from build123d import *

# Parameters (mm, degrees)
BOSS_EXTRUDE1_DEPTH = 3.302


with BuildPart() as part:
    # Sketch2 → Revolve1 (revolve)
    with BuildSketch(Plane(origin=(0, 0, 0), x_dir=(0, 0, -1), z_dir=(1, 0, 0)), mode=Mode.PRIVATE) as revolve1_sk:
        Polygon((0, 3.556), (-4.2672, 3.556), (-4.2672, 5.08), (-7.366, 5.08), (-28.702, 3.8735), (-28.702, 3.556), (-37.7952, 3.33375), (-37.7952, 2.032), (-88.9, 2.032), (-88.9, 0), (0, 0), align=None)
    revolve(revolve1_sk.sketch.rotate(Axis((0, 0, 88.9), (0, 0, -1)), 90), axis=Axis((0, 0, 88.9), (0, 0, -1)))

    # Sketch3 → Boss-Extrude1 (add)
    with BuildSketch(Plane(origin=(0, 0, 4.2672), x_dir=(-1, 0, 0), z_dir=(0, 0, -1))):
        with BuildLine():
            Line((-1.6256, -9.5885), (1.6256, -9.5885))
            ThreePointArc((1.6256, -9.5885), (2.34402049, -9.29092049), (2.6416, -8.5725))
            Line((2.6416, -8.5725), (2.6416, 8.5725))
            ThreePointArc((2.6416, 8.5725), (2.34402049, 9.29092049), (1.6256, 9.5885))
            Line((1.6256, 9.5885), (-1.6256, 9.5885))
            ThreePointArc((-1.6256, 9.5885), (-2.34402049, 9.29092049), (-2.6416, 8.5725))
            Line((-2.6416, 8.5725), (-2.6416, -8.5725))
            ThreePointArc((-2.6416, -8.5725), (-2.34402049, -9.29092049), (-1.6256, -9.5885))
        make_face()
    extrude(amount=BOSS_EXTRUDE1_DEPTH)


solid = part.part
For this review, take the finished solid that the model builds, in its own axes (mm). A direction names the side the tool comes from. Round coordinates to 2 decimals unless told otherwise and drop trailing zeros. Write each loop counter-clockwise with the first axis right and the second up, starting at its lowest first coordinate (ties: lowest second). Pieces come first, ordered by that corner, then holes. Notation, with made-up numbers: (-16.75, 24.25) - (-3.75, 24.25) arc R11 cw to (-3.75, 37.25) - close; hole circle Ø8 at (-21, 37.5). An arc over 180 degrees is marked (long way). Write item = value, one per line. Start each with the question number.
1. Consider section C-C on z = 73. State the section outline as (x, y) points.
2. Consider section D-D on y = -7.75. State the section outline as (x, z) points, plus the area to 3 significant figures.
3. For pin 1 Ø4 at (x, y) = (1, -7) entering from -Z; pin 2 Ø2.5 at (y, z) = (5, 3) entering from -X; pin 3 Ø1.7 at (y, z) = (5, 2) entering from +X, all flat-tipped, find the tip position at first contact; note any pin that passes through.
4. Consider section A-A on y = 0. State the section outline as (x, z) points, plus the area to 3 significant figures.
5. For faces 1 (the face through (-0.661, -5.037, 5.838)), 2 (the face through (-2.822, 2.164, 1.689)), 3 (the face through (2.642, -5, 3)), 4 (the face through (4, 0, 4.267)), 5 (the face through (-4, 0, 4.267)), list the 3-axis set-ups (+Z, -Z, +X, -X, +Y, -Y) from which the entire face can be reached by the end or side of a thin tool; tool diameter is ignored.
6. Consider section B-B on x = 0. State the section outline as (y, z) points, plus the area to 3 significant figures.
7. Wall thickness on L1, parallel to Z at x = -1.5, y = -7.25; L2, parallel to X at y = 0.75, z = 34; L3, parallel to Y at x = -1, z = 58.5: over which ranges is each line inside the solid? List them lowest first.
Evaluation:
q1.outline = circle Ø4.06 at (0, 0)
q2.outline = (-2.64, 0.97) - (2.64, 0.97) - (2.64, 4.27) - (-2.64, 4.27) - close
q2.area = 17.4 mm2
q3.pin_1 = 0.97
q3.pin_2 = -2.64
q3.pin_3 = 2.64
q4.outline = (-5.08, 4.27) - (-3.56, 4.27) - (-3.56, 0) - (3.56, 0) - (3.56, 4.27) - (5.08, 4.27) - (5.08, 7.37) - (3.87, 28.7) - (3.56, 28.7) - (3.33, 37.8) - (2.03, 37.8) - (2.03, 88.9) - (-2.03, 88.9) - (-2.03, 37.8) - (-3.33, 37.8) - (-3.56, 28.7) - (-3.87, 28.7) - (-5.08, 7.37) - close
q4.area = 523 mm2
q5.face_1 = +Z
q5.face_2 = -Z
q5.face_3 = -Z, +X, -Y
q5.face_4 = -Z, +X
q5.face_5 = -Z, -X
q6.outline = (-9.59, 0.97) - (-3.56, 0.97) - (-3.56, 0) - (3.56, 0) - (3.56, 0.97) - (9.59, 0.97) - (9.59, 4.27) - (5.08, 4.27) - (5.08, 7.37) - (3.87, 28.7) - (3.56, 28.7) - (3.33, 37.8) - (2.03, 37.8) - (2.03, 88.9) - (-2.03, 88.9) - (-2.03, 37.8) - (-3.33, 37.8) - (-3.56, 28.7) - (-3.87, 28.7) - (-5.08, 7.37) - (-5.08, 4.27) - (-9.59, 4.27) - close
q6.area = 563 mm2
q7.L1 = 0.97 to 4.27
q7.L2 = -3.34 to 3.34
q7.L3 = -1.77 to 1.77
